```python
from build123d import *

# Parameters (mm, degrees)
F0_W     = 50.8
F0_H     = 19.05
F1_DEPTH = 1111.25
F2_W     = 122.435573
F2_H     = 50.8
F2_W_2   = 93.867282
F2_W_3   = 343.160421
F2_H_2   = 127
F2_W_4   = 239.549167
F3_DEPTH = 25.4
F4_R     = 4.7625
F5_DEPTH = 25.4


with BuildPart() as f1:
    # F0 (on Top) → F1 (new body)
    with BuildSketch(Plane.XY):
        Rectangle(F0_W, F0_H)
    extrude(amount=F1_DEPTH)

    # F2 (on Front) → F3 (cut)
    with BuildSketch(Plane.XZ):
        with Locations((22.446524, 25.4)):
            Rectangle(F2_W, F2_H)
        with Locations((2.720783, 755.65)):
            Rectangle(F2_W_2, F2_H)
        with Locations((-38.781822, 1047.75)):
            Rectangle(F2_W_3, F2_H_2)
        with Locations((-25.794175, 254)):
            Rectangle(F2_W_4, F2_H)
    extrude(amount=F3_DEPTH, mode=Mode.SUBTRACT)

    # F4 (on Front) → F5 (cut)
    with BuildSketch(Plane.XZ):
        with Locations((-15.875, 254)):
            Circle(F4_R)
        with Locations((-15.875, 482.6)):
            Circle(F4_R)
    extrude(amount=F5_DEPTH, mode=Mode.SUBTRACT)


solid = f1.part
```
The model under review builds one solid part; all positions refer to its coordinate system, in mm. A direction names the side the tool comes from. Round coordinates to 2 decimals unless told otherwise and drop trailing zeros. Order: outer loops, then holes, each group sorted by start corner. A loop starts at its lowest first (then second) coordinate and runs counter-clockwise, first axis right, second up. Notation, with made-up numbers: (-28, 33) -> (-17, 33) arc R29 cw to (-17, 70) -> close; hole circle Ø8 at (63.25, 43.5). An arc over 180 degrees is marked (long way). One line per item, written item: value. Start each with the question number.
Q1. Take a section at A-A (x = 2.5). Write out the cut boundary in (y, z) (3 decimals), and give its area (3 significant figures).
Q2. Machinability: for faces 3 (the face through (0, -9.525, 881)), 4 (the face through (0, 0, 26)), 5 (the face through (-25.4, 0, 548)), 6 (the face through (0, 0, 1049)), 7 (the face through (0, 0, 756)), which of the approach directions +Z, -Z, +X, -X, +Y, -Y give a long, thin tool a straight path to every point of the face, cutting with its end or side? Answer none if there is none.
Q3. Clearance check with flat-ended pins moving along their axes: pin 1 Ø15 at (x, z) = (10.5, 14.5) entering from -Y; pin 2 Ø3 at (x, y) = (-5.5, -3.5) entering from -Z; pin 3 Ø3 at (x, y) = (5, -4.5) entering from +Z. State where each tip first meets the part, or that it passes through.
Q4. Mouldability with a two-part tool opening along Z and no side actions: class faces 1 (the face through (0, 0, 254)), 2 (the face through (0, -9.525, 138)) as released by +Z, released by -Z, zero draft, split by the parting line, or undercut.
Q5. Wall thickness on line 1 (Z direction, x = 19.5, y = -2.25); line 2 (X direction, y = -6.75, z = 482.6); line 3 (Y direction, x = 19.5, z = 247) (3 decimals): over which ranges is each line inside the solid? List them lowest first.
Reported:
1. outline: (-9.525, 50.8) -> (0, 50.8) -> (0, 0) -> (9.525, 0) -> (9.525, 1111.25) -> (0, 1111.25) -> (0, 984.25) -> (-9.525, 984.25) -> (-9.525, 781.05) -> (0, 781.05) -> (0, 730.25) -> (-9.525, 730.25) -> (-9.525, 279.4) -> (0, 279.4) -> (0, 228.6) -> (-9.525, 228.6) -> close
1. area: 18,500 mm2
2. face 3: +Z, -Z, +X, -X, -Y
2. face 4: -Z, +X, -X, -Y
2. face 5: +Z, -Z, -X, +Y, -Y
2. face 6: +Z, +X, -X, -Y
2. face 7: +X, -X, -Y
3. pin 1: stops at y = 0
3. pin 2: stops at z = 50.8
3. pin 3: stops at z = 984.25
4. face 1: undercut
4. face 2: zero draft
5. line 1: z = 50.8 to 228.6, 279.4 to 730.25, 781.05 to 984.25
5. line 2: x = -25.4 to -20.64, -11.11 to 25.4
5. line 3: y = 0 to 9.525
